Print and shaded views of the part. All mm, measured from the part's lowest x, y and z. A direction names the side the tool comes from. Round coordinates to 2 decimals unless told otherwise and drop trailing zeros. Write each loop counter-clockwise with the first axis right and the second up, starting at its lowest first coordinate (ties: lowest second). Pieces come first, ordered by that corner, then holes.
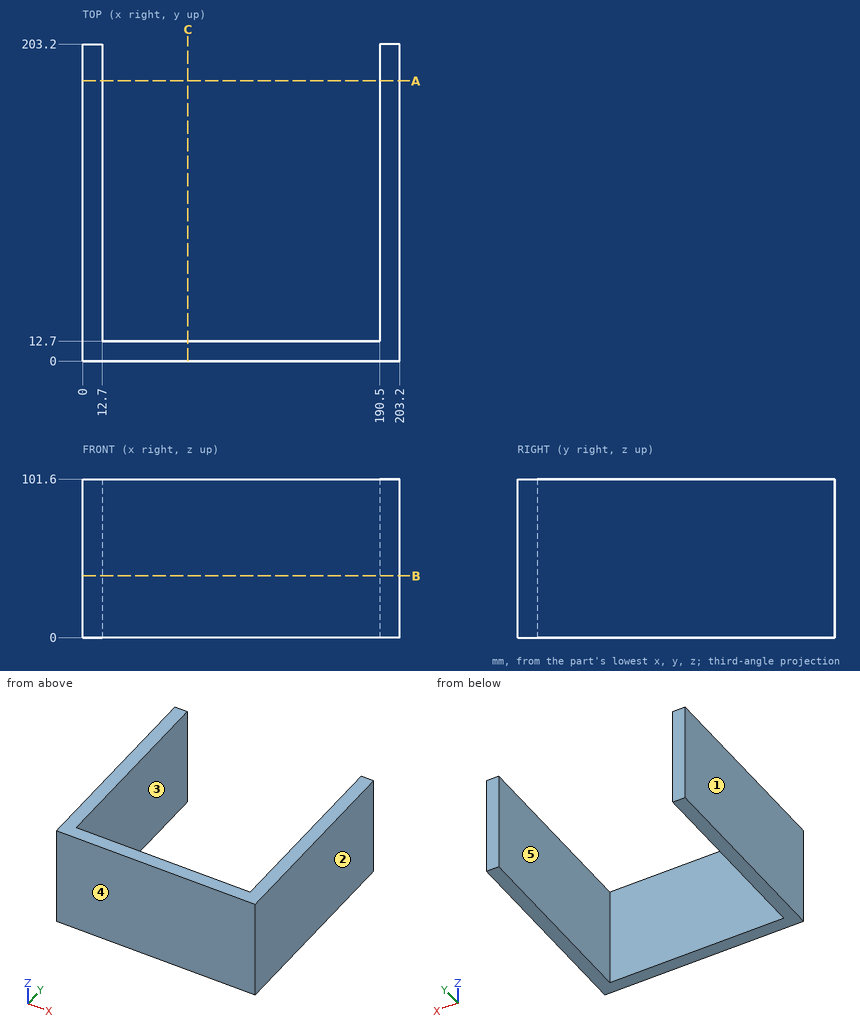
1) Slice it at C-C (x = 67.5). Write the cut outline in (y, z).
Results:
outline: (0, 0) - (12.7, 0) - (12.7, 101.6) - (0, 101.6) - close
2) Wall check: L1, parallel to X at y = 148.5, z = 11.5; L2, parallel to Y at x = 160.5, z = 24. Give the ranges that are in metal, low to high.
Results:
L1: x = 0 to 12.7, 190.5 to 203.2
L2: y = 0 to 12.7
3) Slice it at B-B (z = 39.5). Write the cut outline in (x, y).
Results:
outline: (0, 0) - (203.2, 0) - (203.2, 203.2) - (190.5, 203.2) - (190.5, 12.7) - (12.7, 12.7) - (12.7, 203.2) - (0, 203.2) - close
4) Pin check, flat tip, straight feed: pin 1 Ø6 at (x, z) = (107, 25) entering from +Y. Stop position of the tip, or through.
Results:
pin 1: stops at y = 12.7
5) Mould opens along X. For the marked faces 1, 2 and 3 say: released by +X, released by -X, zero draft, split by the parting line, or undercut.
Results:
face 1: released by -X
face 2: released by +X
face 3: undercut
6) Which spindle directions (+Z, -Z, +X, -X, +Y, -Y) get a long thin tool onto all of the face, cutting with end or side? Do the marked faces 4 and 5. Say none if no direction does.
Results:
face 4: +Z, -Z, +X, -X, -Y
face 5: +Z, -Z, +Y
7) Slice it at A-A (y = 179.5). Write the cut outline in (x, z), plus the area to 3 significant figures.
Results:
outline: (0, 0) - (12.7, 0) - (12.7, 101.6) - (0, 101.6) - close; (190.5, 0) - (203.2, 0) - (203.2, 101.6) - (190.5, 101.6) - close
area: 2,580 mm2
